Geometry check sheet. Reference: the model listing, model coordinates, mm. A direction names the side the tool comes from. Round coordinates to 2 decimals unless told otherwise and drop trailing zeros. Write each loop counter-clockwise with the first axis right and the second up, starting at its lowest first coordinate (ties: lowest second). Pieces come first, ordered by that corner, then holes. Notation, with made-up numbers: M -22,36.25 L -11,36.25 A19 cw -11,47.25 Z; hole C 47.25,22 d4. An arc over 180 degrees is marked long. Put each result on its own line as item: value. Start each with the question number.
(1) Material ranges on probe 1 along X at (y, z) = (2.75, 0) (3 decimals); probe 2 along Y at (x, z) = (15.5, 7); probe 3 along X at (y, z) = (5.25, -1.5), recorded low to high.
(2) Tool access check on faces 1 (the cylindrical face through (17.23, 1.48, -15.9)), 2 (the cylindrical face through (0.33, 8.204, -7.493)). Record the directions out of +Z, -Z, +X, -X, +Y, -Y that give a thin tool (end or side, any length) a straight path to the whole face; none if there is none.
(3) Gauge pin test, flat ends, axial feed: pin 1 (1 mm diameter, centred on x = 14.5, y = 3, fed in from -Z); pin 2 (3.5 mm diameter, centred on x = 15.7, z = -15.7, fed in from +Y); pin 3 (3 mm diameter, centred on x = 0, z = 22.2, fed in from -Y); pin 4 (10 mm diameter, centred on x = -6, z = 12.5, fed in from +Y). Record the tip position at first contact, or that the pin passes through.
(4) Section check C-C on x = -13.5. Record the cut outline in (y, z).
(5) Section check A-A on z = 0. Record the cut outline in (x, y) (3 decimals), then the cut area to 3 significant figures.
(6) Mould release check, pull along X, two halves, no side actions. Record for faces 3 (the cylindrical face through (-17.07, 1.48, 16.41)), 4 (the cylindrical face through (-24.1, 1.5, -5.4)), 5 (the flat face through (12, 3, -7)), 6 (the flat face through (-1.01, 6.95, -2.37)): pulls with the +X half, pulls with the -X half, needs draft (parallel to the pull), parting line crosses it, or undercut.
from build123d import *

# Parameters (mm, degrees)
SKETCH_1_R               = 24.696170665
SKETCH_1_R_2             = 1.55
SKETCH_1_R_3             = 7.5
EXTRUDE_1_DEPTH          = 3
SKETCH_1_4_R             = 7.5
EXTRUDE_2_DEPTH          = 11.5
CHAMFER_2_SIZE           = 2
CUT_EXTRUDE_2_DEPTH      = 40.04942882
CUT_EXTRUDE_2_DEPTH_BACK = 40.04942882
SKETCH_5_R               = 1.55


with BuildPart() as part:
    # Sketch 1 → Extrude 1 (new body)
    with BuildSketch(Plane(origin=(0, 0, 0), x_dir=(1, 0, 0), z_dir=(0, 1, 0))):
        with Locations(Location((0, 0, 0), (0, 0, 270))):
            Circle(SKETCH_1_R)
        with Locations(Location((-22.196170665, 0, 0), (0, 0, 270))):
            Circle(SKETCH_1_R_2, mode=Mode.SUBTRACT)
        with Locations(Location((-15.695062794, 15.695062794, 0), (0, 0, 270))):
            Circle(SKETCH_1_R_2, mode=Mode.SUBTRACT)
        with Locations(Location((0, 22.196170665, 0), (0, 0, 270))):
            Circle(SKETCH_1_R_2, mode=Mode.SUBTRACT)
        with Locations(Location((15.695062794, 15.695062794, 0), (0, 0, 270))):
            Circle(SKETCH_1_R_2, mode=Mode.SUBTRACT)
        with Locations(Location((22.196170665, 0, 0), (0, 0, 270))):
            Circle(SKETCH_1_R_2, mode=Mode.SUBTRACT)
        with Locations(Location((15.695062794, -15.695062794, 0), (0, 0, 270))):
            Circle(SKETCH_1_R_2, mode=Mode.SUBTRACT)
        with Locations(Location((0, -22.196170665, 0), (0, 0, 270))):
            Circle(SKETCH_1_R_2, mode=Mode.SUBTRACT)
        with Locations(Location((-15.695062794, -15.695062794, 0), (0, 0, 270))):
            Circle(SKETCH_1_R_2, mode=Mode.SUBTRACT)
        with Locations(Location((0, 0, 0), (0, 0, 270))):
            Circle(SKETCH_1_R_3, mode=Mode.SUBTRACT)
    extrude(amount=EXTRUDE_1_DEPTH)

    # Sketch 1_4 → Extrude 2 (add)
    with BuildSketch(Plane(origin=(0, 0, 0), x_dir=(1, 0, 0), z_dir=(0, 1, 0))):
        with Locations(Location((0, 0, 0), (0, 0, 270))):
            Circle(SKETCH_1_4_R)
        with BuildLine():
            Line((-2.452023129, 1.77149868), (0.481203452, 2.986480912))
            ThreePointArc((0.481203452, 2.986480912), (1.157617383, -2.794735586), (-2.452023129, 1.77149868))
        make_face(mode=Mode.SUBTRACT)
    extrude(amount=EXTRUDE_2_DEPTH)

    # Chamfer 2
    chamfer_2_edges = [part.edges().sort_by_distance(p)[0] for p in [
        (0, 3, -7.5),
    ]]
    chamfer(chamfer_2_edges, length=CHAMFER_2_SIZE)

    # Sketch 5 → Cut-Extrude 2 (cut, two sides: drawn at the far end of the back side and taken through both)
    with BuildSketch(Plane(origin=(-0.985409838, 0, -2.378989796), x_dir=(0.9238795325112868, 0, -0.38268343236508967), z_dir=(0.3826834323650896, 0, 0.9238795325112867)).offset(-CUT_EXTRUDE_2_DEPTH_BACK)):
        with Locations(Location((0, 2.5, 0), (0, 0, 341.181195654))):
            Circle(SKETCH_5_R)
    extrude(amount=CUT_EXTRUDE_2_DEPTH + CUT_EXTRUDE_2_DEPTH_BACK, mode=Mode.SUBTRACT)


solid = part.part
Answers follow:
1. probe 1: x = -24.696 to -23.746, -20.646 to -3.025, 3.025 to 20.646, 23.746 to 24.696
1. probe 2: y = 0 to 3
1. probe 3: x = -7.35 to -2.63, 2.63 to 7.35
2. face 1: +Y, -Y
2. face 2: +Y
3. pin 1: stops at z = -20.34
3. pin 2: stops at y = 3
3. pin 3: passes through
3. pin 4: stops at y = 3.63
4. outline: M 0,-20.68 L 3,-20.68 L 3,20.68 L 0,20.68 Z
5. outline: M -24.696,0 L -23.746,0 L -23.746,3 L -24.696,3 Z; M -20.646,0 L -3.025,0 L -3.025,11.5 L -7.5,11.5 L -7.5,5 L -9.5,3 L -20.646,3 Z; M 3.025,0 L 20.646,0 L 20.646,3 L 9.5,3 L 7.5,5 L 7.5,11.5 L 3.025,11.5 Z; M 23.746,0 L 24.696,0 L 24.696,3 L 23.746,3 Z
5. area: 192 mm^2
6. face 3: undercut
6. face 4: parting line crosses it
6. face 5: needs draft
6. face 6: undercut
